Build history of the part. All positions in model axes, mm. Face numbers are marked on the shaded views. A direction names the side the tool comes from. Coordinates: 2 decimals unless noted, no trailing zeros. Order: outer loops, then holes, each group sorted by start corner. A loop starts at its lowest first (then second) coordinate and runs counter-clockwise, first axis right, second up. Notation, with made-up numbers: (-2.75, 50) - (51.25, 50) arc R15 cw to (51.25, 54) - close; hole circle Ø1 at (72, 24). An arc over 180 degrees is marked (long way). One line per item, written item: value.
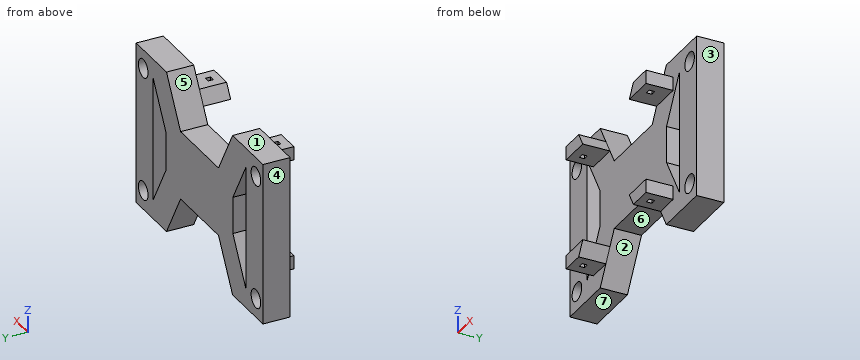
from build123d import *

# Parameters (mm, degrees)
SKETCH003_R  = 3.4
PAD001_DEPTH = 10
PAD002_DEPTH = 10
SKETCH005_W  = 2
SKETCH005_H  = 2
POCKET_DEPTH = 53.001


with BuildPart() as part:
    # Sketch003 → Pad001 (new body)
    with BuildSketch(Plane.XZ):
        Polygon((0, 60), (21.539201, 60), (31.540737, 42.676832), (58.459263, 42.676832), (68.460799, 60), (90, 60), (90, 0), (68.460799, 0), (58.459263, 17.323168), (31.540737, 17.323168), (21.539201, 0), (0, 0), align=None)
        with Locations((5, 53)):
            Circle(SKETCH003_R, mode=Mode.SUBTRACT)
        with Locations((5, 7)):
            Circle(SKETCH003_R, mode=Mode.SUBTRACT)
        with Locations((85, 7)):
            Circle(SKETCH003_R, mode=Mode.SUBTRACT)
        with Locations((85, 53)):
            Circle(SKETCH003_R, mode=Mode.SUBTRACT)
        Polygon((78, 53), (68.649322, 36.80415), (68.649322, 23.19585), (78, 7), align=None, mode=Mode.SUBTRACT)
        Polygon((12, 53), (12, 7), (21.350678, 23.19585), (21.350678, 36.80415), align=None, mode=Mode.SUBTRACT)
    extrude(amount=PAD001_DEPTH)

    # Sketch004 (on Face26 of Pad001) → Pad002 (join)
    with BuildSketch(Plane.XZ.offset(10)):
        Polygon((16.675339, 53), (25.580653, 53), (28.467405, 48), (16.675339, 48), align=None)
        Polygon((64.419347, 53), (73.324661, 53), (73.324661, 48), (61.532595, 48), align=None)
        Polygon((16.675339, 12), (16.675339, 7), (25.580653, 7), (28.467405, 12), align=None)
        Polygon((73.324661, 12), (61.532595, 12), (64.419347, 7), (73.324661, 7), align=None)
    extrude(amount=PAD002_DEPTH)

    # Sketch005 (on Face39 of Pad002) → Pocket (cut, through all)
    with BuildSketch(Plane(origin=(0, 0, 53), x_dir=(-1, 0, 0), z_dir=(0, 0, 1))):
        with Locations((-21.127996, 16)):
            Rectangle(SKETCH005_W, SKETCH005_H)
        with Locations((-68.872004, 16)):
            Rectangle(SKETCH005_W, SKETCH005_H)
    extrude(amount=-POCKET_DEPTH, mode=Mode.SUBTRACT)


solid = part.part
1. 3-axis set-ups, long thin cutter, end or side, ignore diameter. For the marked faces 5, 6 and 7: which of +Z, -Z, +X, -X, +Y, -Y reach the whole face in a straight line?
Values found:
face 5: +Z, +Y, -Y
face 6: -Z, +Y, -Y
face 7: -Z, +X, -X, +Y, -Y
2. Flat gauge pins, fed straight in: P1, Ø1, axis at y = -16, z = 49.5, coming from the +X side; P2, Ø4.5, axis at x = 66.5, y = -14, coming from the -Z side; P3, Ø8, axis at x = 14.5, y = -15, coming from the +Z side. Where does each tip first touch, or does it go through?
Values found:
P1: stops at x = 73.32
P2: stops at z = 7
P3: stops at z = 53
3. Band-saw the part on A-A, the plane y = -13.25. Give the cut face in (x, z), and give its area (3 significant figures).
Values found:
outline: (16.68, 7) - (25.58, 7) - (28.47, 12) - (16.68, 12) - close; (16.68, 48) - (28.47, 48) - (25.58, 53) - (16.68, 53) - close; (61.53, 12) - (64.42, 7) - (73.32, 7) - (73.32, 12) - close; (61.53, 48) - (73.32, 48) - (73.32, 53) - (64.42, 53) - close
area: 207 mm2
4. Band-saw the part on B-B, the plane z = 25. Give the cut face in (x, y), and give its area (3 significant figures).
Values found:
outline: (0, -10) - (12, -10) - (12, 0) - (0, 0) - close; (21.35, -10) - (68.65, -10) - (68.65, 0) - (21.35, 0) - close; (78, -10) - (90, -10) - (90, 0) - (78, 0) - close
area: 713 mm2
5. Probe line 1 along Z through (x, y) = (85, -8); line 2 along X through (y, z) = (-5, 32); line 3 along Z through (x, y) = (17, -10.5). List the from-to ranges inside material, lowest first.
Values found:
line 1: z = 0 to 3.6, 10.4 to 49.6, 56.4 to 60
line 2: x = 0 to 12, 21.35 to 68.65, 78 to 90
line 3: z = 7 to 12, 48 to 53
6. Band-saw the part on D-D, the plane y = -3.75. Give the cut face in (x, z).
Values found:
outline: (0, 0) - (21.54, 0) - (31.54, 17.32) - (58.46, 17.32) - (68.46, 0) - (90, 0) - (90, 60) - (68.46, 60) - (58.46, 42.68) - (31.54, 42.68) - (21.54, 60) - (0, 60) - close; hole circle Ø6.8 at (5, 7); hole circle Ø6.8 at (5, 53); hole (12, 7) - (21.35, 23.2) - (21.35, 36.8) - (12, 53) - close; hole (68.65, 23.2) - (78, 7) - (78, 53) - (68.65, 36.8) - close; hole circle Ø6.8 at (85, 7); hole circle Ø6.8 at (85, 53)
7. Two-plate mould, pull along X, no slides. Class the marked faces 1, 2, 3 and 4: pulls with the +X half, pulls with the -X half, needs draft (parallel to the pull), parting line crosses it, or undercut.
Values found:
face 1: needs draft
face 2: undercut
face 3: pulls with the +X half
face 4: pulls with the -X half
8. Band-saw the part on C-C, the plane x = 85. Give the cut face in (y, z).
Values found:
outline: (-10, 0) - (0, 0) - (0, 3.6) - (-10, 3.6) - close; (-10, 10.4) - (0, 10.4) - (0, 49.6) - (-10, 49.6) - close; (-10, 56.4) - (0, 56.4) - (0, 60) - (-10, 60) - close
